Could you check a few things on this model? Use its own coordinates, in mm. Face numbers are marked on the shaded views. Give positions to 0.01 mm unless a question says otherwise; leave off trailing zeros. Order: outer loops, then holes, each group sorted by start corner. A loop starts at its lowest first (then second) coordinate and runs counter-clockwise, first axis right, second up.
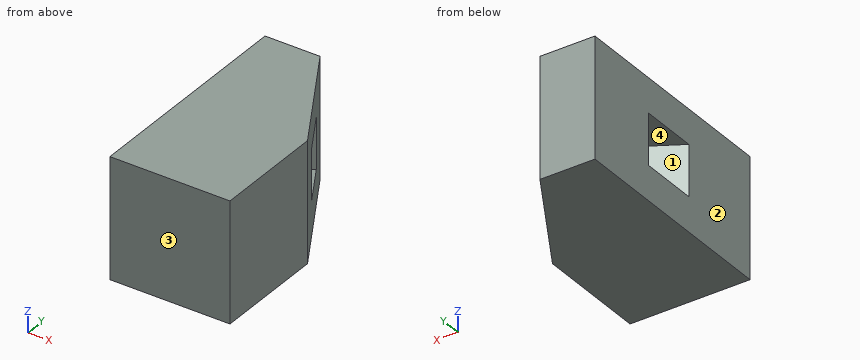
from build123d import *

# Parameters (mm, degrees)
SKETCH_1_W          = 8
SKETCH_1_H          = 8
EXTRUDE_1_DEPTH     = 15
CUT_EXTRUDE_1_REACH = 20.788
SKETCH_3_W          = 3.4
SKETCH_3_H          = 3.4
CUT_EXTRUDE_2_DEPTH = 10


with BuildPart() as part:
    # 草图1 → 凸台-拉伸1 (new body)
    with BuildSketch(Plane(origin=(0, 0, 0), x_dir=(1, 0, 0), z_dir=(0, 1, 0))):
        with Locations((4, 4)):
            Rectangle(SKETCH_1_W, SKETCH_1_H)
    extrude(amount=EXTRUDE_1_DEPTH)

    # 草图2 → 切除-拉伸1 (cut, up to next)
    with BuildSketch(Plane(origin=(0, 0, -8), x_dir=(-1, 0, 0), z_dir=(0, 0, -1)), mode=Mode.PRIVATE) as cut_extrude_1_sk1:
        Polygon((-8, 7.5), (-3.669872981, 15), (-8, 15), align=None)
    cut_extrude_1_tool1 = extrude(cut_extrude_1_sk1.sketch, amount=-CUT_EXTRUDE_1_REACH, mode=Mode.PRIVATE) & part.part
    add(cut_extrude_1_tool1.solids().sort_by_distance((6.556624, 12.5, -8))[0], mode=Mode.SUBTRACT)

    # 草图3 → 切除-拉伸2 (cut)
    with BuildSketch(Plane(origin=(9.247595264, 5.339101615, 0), x_dir=(0, 0, -1), z_dir=(0.8660254037844417, 0.4999999999999948, 0))):
        with Locations((4, 6.825317547)):
            Rectangle(SKETCH_3_W, SKETCH_3_H)
    extrude(amount=-CUT_EXTRUDE_2_DEPTH, mode=Mode.SUBTRACT)


solid = part.part
Item 1: Imagine slicing it at B-B on x = 4.75. List the corners of the cut face in (y, z) for me.
Findings:
outline: (0, -8) - (13.13, -8) - (13.13, 0) - (0, 0) - close; hole (8.66, -5.7) - (12.59, -5.7) - (12.59, -2.3) - (8.66, -2.3) - close
Item 2: Imagine slicing it at A-A on z = -5. List the corners of the cut face in (x, y) for me, then the cut area to 3 significant figures.
Findings:
outline: (0, 0) - (8, 0) - (8, 7.5) - (6.68, 9.78) - (0, 5.92) - close; (0, 9.84) - (4.98, 12.72) - (3.67, 15) - (0, 15) - close
area: 80.9 mm2
Item 3: We'd pull the mould along Y, two halves only. Please class the marked faces 1, 2, 3 and 4: +Y half, -Y half, draft (parallel to the pull), parting line (faces both ways), or undercut.
Findings:
face 1: undercut
face 2: draft
face 3: -Y half
face 4: undercut
Item 4: Please list where these lines run through material, in increasing order: line 1 along Z through (x, y) = (2, 7.75); line 2 along Y through (x, z) = (1.5, -3.25); line 3 along Y through (x, z) = (1.75, -5).
Findings:
line 1: z = -8 to -5.7, -2.3 to 0
line 2: y = 0 to 6.78, 10.71 to 15
line 3: y = 0 to 6.93, 10.85 to 15
Item 5: Imagine slicing it at C-C on y = 11.5. List the corners of the cut face in (x, z) for me, then the cut area to 3 significant figures.
Findings:
outline: (0, -8) - (5.69, -8) - (5.69, -5.7) - (2.87, -5.7) - (2.87, -2.3) - (5.69, -2.3) - (5.69, 0) - (0, 0) - close
area: 35.9 mm2
Item 6: Imagine slicing it at D-D on x = 6.25. List the corners of the cut face in (y, z) for me.
Findings:
outline: (0, -8) - (10.53, -8) - (10.53, -5.7) - (9.53, -5.7) - (9.53, -2.3) - (10.53, -2.3) - (10.53, 0) - (0, 0) - close
